Input: dimensioned drawing with shaded views. Units: mm. Origin: part minimum x, y, z. Give positions to 0.01 mm unless a question says otherwise; leave off trailing zeros. Loops run counter-clockwise (first coordinate to the right, second up) from the corner with the lowest first, then second, coordinate; pieces in that order, holes last. Notation, with made-up numbers: M 49.25,80.5 L 71.25,80.5 A7 cw 71.25,84.5 Z; hole C 76,29 d1. An arc over 180 degrees is marked long. One line per question, with ' | ' between items. Start each with the question number.
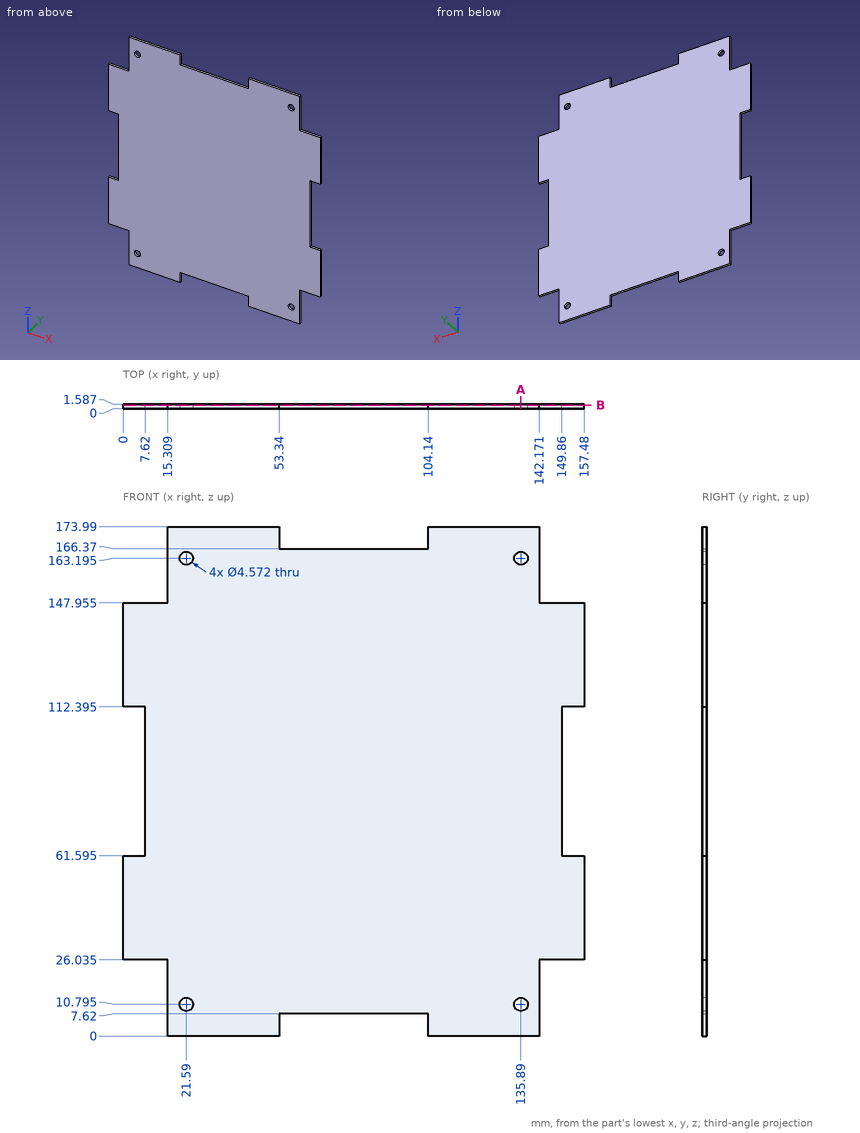
Q1. Contact query for flat-ended pins moving along their axis: pin 1 (3.5 mm diameter, centred on x = 135.89, z = 163.195, fed in from +Y); pin 2 (0.8 mm diameter, centred on x = 10.5, y = 0.5, fed in from -Z) (1 decimal); pin 3 (0.5 mm diameter, centred on x = 152.5, y = 0.5, fed in from +Z) (1 decimal); pin 4 (0.5 mm diameter, centred on y = 0.5, z = 14.5, fed in from +X). Output: stop coordinate, or through.
Q2. Section A-A, the plane x = 135.89. Output: boundary loops of the cut face in (y, z).
Q3. Material intervals for L1, parallel to Z at x = 135.89, y = 0.45; L2, parallel to Z at x = 60, y = 0.7; L3, parallel to X at y = 1.5, z = 62, sorted ascending.
Q4. Section B-B, the plane y = 1.2. Count the separate pieces of the cut face and the enclosed holes in it, plus the area to 3 significant figures.
Model answer:
1) pin 1: passes through | pin 2: stops at z = 26 | pin 3: stops at z = 148 | pin 4: stops at x = 142.17
2) outline: M 0,0 L 1.59,0 L 1.59,8.51 L 0,8.51 Z; M 0,13.08 L 1.59,13.08 L 1.59,160.91 L 0,160.91 Z; M 0,165.48 L 1.59,165.48 L 1.59,173.99 L 0,173.99 Z
3) L1: z = 0 to 8.51, 13.08 to 160.91, 165.48 to 173.99 | L2: z = 7.62 to 166.37 | L3: x = 7.62 to 149.86
4) separate pieces: 1 | enclosed holes: 4 | area: 24,200 mm^2
